Work out the finished part from the listing and answer in its coordinate system (mm). Face numbers are marked on the shaded views. Give positions to 0.01 mm unless a question says otherwise; leave off trailing zeros. Order: outer loops, then holes, each group sorted by start corner. A loop starts at its lowest first (then second) coordinate and runs counter-clockwise, first axis right, second up. Notation, with made-up numbers: M -0.5,19 L 25.5,19 A13 cw 25.5,41 Z; hole C 35.25,42 d3. An arc over 180 degrees is marked long. One line per item, written item: value.
from build123d import *

# Parameters (mm, degrees)
EXTRUDE_1_DEPTH     = 140
CUT_EXTRUDE_1_DEPTH = 4
CUT_EXTRUDE_2_DEPTH = 11
SKETCH_4_R          = 6
CUT_EXTRUDE_3_DEPTH = 11
SKETCH_5_W          = 14
SKETCH_5_H          = 136
EXTRUDE_2_DEPTH     = 1
FILLET_1_R          = 2


with BuildPart() as part:
    # Эскиз1 → Бобышка-Вытянуть1 (new body)
    with BuildSketch(Plane.XY):
        Polygon((-28, 0), (28, 0), (28, 2), (24, 8.92820323), (24, 10), (-24, 10), (-24, 8.92820323), (-28, 2), align=None)
    extrude(amount=EXTRUDE_1_DEPTH)

    # Эскиз2 → Вырез-Вытянуть1 (cut)
    with BuildSketch(Plane.XZ):
        Polygon((-22, 140), (-22, 131), (-17, 116), (-17, 112), (-21, 112), (-21, 28), (-17, 28), (-17, 24), (-22, 9), (-22, 0), (22, 0), (22, 9), (17, 24), (17, 28), (21, 28), (21, 112), (17, 112), (17, 116), (22, 131), (22, 140), align=None)
    extrude(amount=-CUT_EXTRUDE_1_DEPTH, mode=Mode.SUBTRACT)

    # Эскиз3 → Вырез-Вытянуть2 (cut, through all)
    with BuildSketch(Plane(origin=(0, 10, 0), x_dir=(1, 0, 0), z_dir=(0, 1, 0))):
        with BuildLine():
            Line((2.75, -20), (2.75, -94))
            ThreePointArc((2.75, -94), (0, -96.75), (-2.75, -94))
            Line((-2.75, -94), (-2.75, -20))
            ThreePointArc((-2.75, -20), (0, -17.25), (2.75, -20))
        make_face()
    extrude(amount=-CUT_EXTRUDE_2_DEPTH, mode=Mode.SUBTRACT)

    # Эскиз4 → Вырез-Вытянуть3 (cut, through all)
    with BuildSketch(Plane(origin=(0, 10, 0), x_dir=(1, 0, 0), z_dir=(0, 1, 0))):
        with Locations((0, -20)):
            Circle(SKETCH_4_R)
    extrude(amount=-CUT_EXTRUDE_3_DEPTH, mode=Mode.SUBTRACT)

    # Эскиз5 → Бобышка-Вытянуть2 (add)
    with BuildSketch(Plane(origin=(0, 10, 0), x_dir=(1, 0, 0), z_dir=(0, 1, 0))):
        with Locations((15, -70)):
            Rectangle(SKETCH_5_W, SKETCH_5_H)
        with Locations((-15, -70)):
            Rectangle(SKETCH_5_W, SKETCH_5_H)
    extrude(amount=EXTRUDE_2_DEPTH)

    # Скругление1
    fillet_1_edges = [part.edges().sort_by_distance(p)[0] for p in [
        (2.75, 7, 25.332682252),
        (-8, 10.5, 138),
        (-8, 10.5, 2),
        (-22, 10.5, 2),
        (-22, 10.5, 138),
        (22, 10.5, 138),
        (22, 10.5, 2),
        (8, 10.5, 2),
        (8, 10.5, 138),
        (-2.75, 7, 25.332682252),
    ]]
    fillet(fillet_1_edges, radius=FILLET_1_R)


solid = part.part
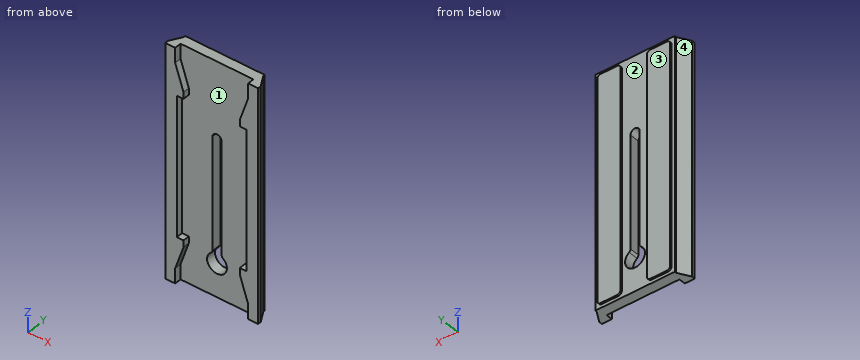
(1) Section A-A, the plane x = 0 is taken. Give the vertices of the cut face in (y, z).
Findings:
outline: M 4,0 L 10,0 L 10,14 L 4,14 Z; M 4,96.75 L 10,96.75 L 10,140 L 4,140 Z
(2) Given P1, Ø0.8, axis at y = 10.5, z = 58.5, coming from the +X side; P2, Ø0.8, axis at x = 13, y = 10.5, coming from the -Z side; P3, Ø1, axis at y = 4.5, z = 98.5, coming from the +X side, each flat-ended and moving along its own axis, determine where each tip first touches the part or whether it passes through.
Findings:
P1: stops at x = 22
P2: stops at z = 2
P3: stops at x = 26.85
(3) Find the intervals of material crossed by probe 1 along Z at (x, y) = (0, 5.3); probe 2 along Y at (x, z) = (-23, 39); probe 3 along X at (y, z) = (8, 55), in increasing order. Write a range as from..to.
Findings:
probe 1: z = 0..14, 96.75..140
probe 2: y = 0..10
probe 3: x = -24.54..-2.75, 2.75..24.54
(4) Section C-C, the plane x = 13 is taken. Give the vertices of the cut face in (y, z).
Findings:
outline: M 4,0 L 10,0 L 10,2 L 11,2 L 11,138 L 10,138 L 10,140 L 4,140 Z
(5) Section D-D, the plane y = 6 is taken. Give the vertices of the cut face in (x, z).
Findings:
outline: M -25.69,0 L 25.69,0 L 25.69,140 L -25.69,140 Z; hole M -3.56,24.83 A6 ccw long 3.56,24.83 A2 cw 2.75,26.44 L 2.75,94 A2.75 ccw -2.75,94 L -2.75,26.44 A2 cw Z
(6) Section B-B, the plane z = 52.5 is taken. Give the vertices of the cut face in (x, y).
Findings:
outline: M -28,0 L -21,0 L -21,4 L -2.75,4 L -2.75,10 L -8,10 L -8,11 L -22,11 L -22,10 L -24,10 L -24,8.93 L -28,2 Z; M 2.75,4 L 21,4 L 21,0 L 28,0 L 28,2 L 24,8.93 L 24,10 L 22,10 L 22,11 L 8,11 L 8,10 L 2.75,10 Z
(7) Determine the mould class of the marked faces 1, 2, 3 and 4 for opening direction X: pulls with the +X half, pulls with the -X half, needs draft (parallel to the pull), parting line crosses it, or undercut.
Findings:
face 1: undercut
face 2: undercut
face 3: needs draft
face 4: pulls with the -X half
